Input: part model. Units: mm. Frame: model coordinates. Face numbers are marked on the shaded views. A direction names the side the tool comes from. Round coordinates to 2 decimals unless told otherwise and drop trailing zeros. Loops run counter-clockwise (first coordinate to the right, second up) from the corner with the lowest first, then second, coordinate; pieces in that order, holes last. Notation, with made-up numbers: M 13.5,42.5 L 38.5,42.5 A16 ccw 38.5,67.5 Z; hole C 68.5,-18.5 d9. An arc over 180 degrees is marked long. Return JSON: item names as keys, results as strings. Group by question number.
1) Section A-A (x = 62.5). Output: boundary loops of the cut face in (y, z).
2) Section D-D (x = 96). Output: boundary loops of the cut face in (y, z).
3) Section B-B (y = 24.5). Output: boundary loops of the cut face in (x, z).
4) Access query for the marked faces 1, 2, 3, 4 and 5. Directions: +Z, -Z, +X, -X, +Y, -Y. A direction counts if a zero-diameter tool reaches every point of the face in a straight line with its end or side. Return the directions, or none.
5) Material intervals for line 1 (X direction, y = 26, z = 10); line 2 (Z direction, x = 25, y = 32); line 3 (X direction, y = 9.5, z = 17), sorted ascending. Write a range as from..to.
6) Mould query, pull axis Y, two halves, no side actions, for the marked faces 6, 7 and 8. Classes: +Y half, -Y half, draft (parallel to the pull), parting line (faces both ways), or undercut.
7) Contact query for flat-ended pins moving along their axis: P1, Ø8, axis at x = 125, z = 10, coming from the +Y side; P2, Ø3, axis at x = 144.5, z = 9.5, coming from the -Y side; P3, Ø5, axis at x = 73.5, y = 29, coming from the -Z side; P4, Ø6, axis at x = 76.5, z = 7, coming from the +Y side. Output: stop coordinate, or through.
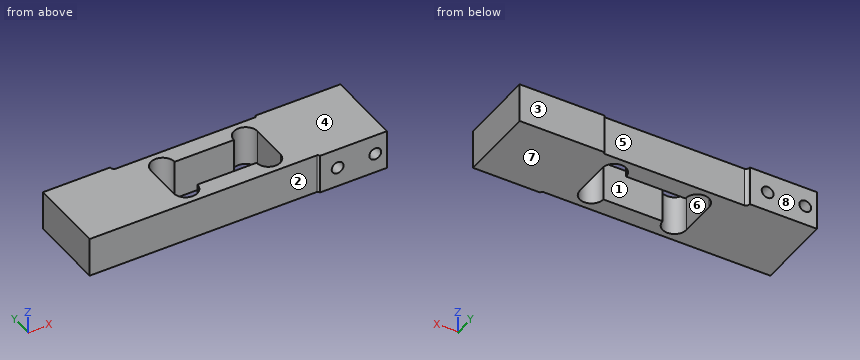
Autodesk Inventor part; units mm, degrees
ref_plane "YZ Plane" through (0, 0, 0) normal (1, 0, 0) x (0, 1, 0)
ref_plane "XZ Plane" through (0, 0, 0) normal (0, 1, 0) x (-1, 0, 0)
ref_plane "XY Plane" through (0, 0, 0) normal (0, 0, 1) x (1, 0, 0)
sketch "Sketch1" plane through (0, 0, 0) normal (0, 0, 1) x (1, 0, 0)
  line L0 (0, 0) -> (150, 0) construction
  line L1 (150, 0) -> (150, 39) construction
  line L2 (150, 39) -> (0, 39) construction
  line L3 (0, 38) -> (150, 38) construction
  line L4 (0, 37) -> (150, 37) construction
  arc A0 (106.25, 37) -> (107, 38) centre (106.0005, 37.9684) ccw
  arc A1 (34, 39) -> (35.5, 37) centre (35.999, 38.9367) ccw
  line L5 (0, -1) -> (150, -1) construction
  arc A2 (116, -1) -> (115.25, 0) centre (115.0005, -0.9684) ccw
  line L6 (75, 37) -> (75, 0) construction
  line L7 (0, 18.5) -> (150, 18.5) construction
  line L8 (75, 28) -> (60, 28)
  arc A3 (60, 28) -> (48, 28) centre (54, 28) ccw
  line L9 (48, 28) -> (48, 18.5)
  line L10 (75, 28) -> (90, 28)
  arc A4 (102, 28) -> (90, 28) centre (96, 28) ccw
  line L11 (102, 28) -> (102, 18.5)
  line L12 (75, 9) -> (60, 9)
  arc A5 (48, 9) -> (60, 9) centre (54, 9) ccw
  line L13 (48, 9) -> (48, 18.5)
  arc A6 (90, 9) -> (102, 9) centre (96, 9) ccw
  line L14 (75, 9) -> (90, 9)
  line L15 (102, 9) -> (102, 18.5)
  line L16 (0, 39) -> (0, 0)
  line L17 (115.25, 0) -> (0, 0)
  line L18 (116, -1) -> (150, -1)
  line L19 (150, -1) -> (150, 38)
  line L20 (150, 38) -> (107, 38)
  line L21 (106.25, 37) -> (35.5, 37)
  line L22 (34, 39) -> (0, 39)
  dimension "d0" = 150
  dimension "d1" = 39
  dimension "d9" = 34
  dimension "d11" = 1
  dimension "d17" = 1
  dimension "d18" = 43
  dimension "d19" = 1.25
  dimension "d20" = 1
  dimension "d21" = 2.5
  dimension "d22" = 2
  dimension "d23" = 1
  dimension "d24" = 34
  dimension "d25" = 1.25
  dimension "d26" = 1
  dimension "d27" = 15
  dimension "d29" = 12
  dimension "d30" = 6
extrude "Extrusion1" add sketch "Sketch1" along normal blind 20
sketch "Sketch2" plane through (116, -1, 0) normal (0, -1, 0) x (1, 0, 0)
  line L0 (0, 20) -> (34, 20) construction
  line L1 (0, 0) -> (34, 0) construction
  line L2 (34, 0) -> (34, 20) construction
  line L3 (34, 20) -> (0, 20) construction
  line L4 (0, 20) -> (0, 0) construction
  circle A0 centre (9, 10) radius 3
  circle A1 centre (28.05, 10) radius 3
  line L5 (-116, 0) -> (-116, 20) construction
  line L6 (34, 0) -> (0, 0) construction
  line L7 (-116, 20) -> (34, 20) construction
  line L8 (34, 20) -> (34, 0) construction
  line L9 (34, 0) -> (-116, 0) construction
  line L10 (-116, 0) -> (-116, 20) construction
  line L11 (-116, 20) -> (-0.75, 20) construction
  dimension "d33" = 6
  dimension "d34" = 10
  dimension "d35" = 25
  dimension "d36" = 6
  dimension "d37" = 19.05
extrude "Extrusion4" cut sketch "Sketch2" against normal blind 18
sketch "Sketch3" plane through (0, 39, 0) normal (0, 1, 0) x (1, 0, 0)
  line L0 (150, 0) -> (150, -20) construction
  line L1 (0, 0) -> (150, 0) construction
  line L2 (150, 0) -> (150, -20) construction
  line L3 (150, -20) -> (0, -20) construction
  line L4 (0, -20) -> (0, 0) construction
  circle A0 centre (5.95, -10) radius 3
  circle A1 centre (25, -10) radius 3
  dimension "d45" = 6
  dimension "d46" = 6
  dimension "d47" = 19.05
  dimension "d51" = 125
  dimension "d52" = 10
  dimension "d53" = 10
extrude "Extrusion5" cut sketch "Sketch3" against normal blind 18
thread "Thread1"
thread "Thread2"
thread "Thread3"
thread "Thread4"
equation "\"d0\" = lcl"
equation "\"d1\" = lch1"
equation "\"d9\" = lcwd2"
equation "\"d11\" = lch2 - lch1"
equation "\"d17\" = lch2 - lch1"
equation "\"d18\" = lcwd3"
equation "\"d23\" = lch2 - lch1"
equation "\"d24\" = lcwd2"
equation "\"d31\" = lcw"
equation "\"d33\" = dia1"
equation "\"d34\" = 0.5 * lcw"
equation "\"d35\" = lcwd1"
equation "\"d36\" = dia1"
equation "\"d37\" = lcsd"
equation "\"d43\" = td"
equation "\"d45\" = d48"
equation "\"d46\" = d48"
equation "\"d47\" = d49"
equation "\"d51\" = lcl - lcwd1"
equation "\"d52\" = 0.5 * lcw"
equation "\"d53\" = 0.5 * lcw"
equation "\"d54\" = td"
equation "\"dias\" = 8.8"
equation "\"stra1\" = 9.5"
equation "\"diab2\" = 6"
equation "\"stra\" = 25"
equation "\"db1\" = 6"
equation "\"ds1\" = 5.8"
equation "\"ds2\" = 1.6"
equation "\"ang\" = 120deg"
equation "\"db2\" = 3"
equation "\"diab3\" = 7"
equation "\"diab4\" = 3"
equation "\"dias1\" = 13.4375"
equation "\"dias3\" = 2"
equation "\"dias4\" = 4"
equation "\"t1\" = 3"
equation "\"t2\" = 3"
equation "\"t3\" = 6"
equation "\"t4\" = 6"
equation "\"t5\" = 3"
equation "\"diab1\" = 19"
equation "\"afw\" = 0.2"
equation "\"lcsd\" = 19.05"
equation "\"lcwd1\" = 25"
equation "\"lcwd2\" = 34"
equation "\"lcw\" = 20"
equation "\"lch1\" = 39"
equation "\"lch2\" = 40"
equation "\"lcl\" = 150"
equation "\"lcwd3\" = 43"
equation "\"dia1\" = 6"
equation "\"td\" = 18"
equation "\"d48\" = 6"
equation "\"d49\" = 19.05"
equation "\"bhh\" = 6"
equation "\"sw\" = 25"
equation "\"spacert\" = 2"
equation "\"sh\" = 31"
equation "\"pvct\" = 5"
equation "\"dia3\" = 8"
equation "\"dia4\" = 11"
equation "\"tankl\" = 379"
equation "\"play\" = 9"
equation "\"holeh\" = 26"
equation "\"surroundt\" = 5"
equation "\"slack\" = 0.5"
equation "\"play2\" = 3"
equation "\"diaoverflow\" = 25"
equation "\"diaph\" = 32"
equation "\"diawater\" = 25"
equation "\"diacucl\" = 32"
equation "\"diaair\" = 32"
equation "\"diasurroundhole\" = 42"
equation "\"diagrate\" = 12"
equation "\"gratespacing\" = 12.02082"
equation "\"bottomdist\" = 9.6355"
equation "\"sidedist\" = 13.9375"
equation "\"diahcl\" = 32"
equation "\"bracketwtop\" = 6"
equation "\"bracketwbottom\" = 6"
equation "\"nett\" = 1"
equation "\"nethole\" = 16"
equation "\"netside\" = 3.5"
equation "\"nettop\" = 7"
equation "\"netholespacing\" = 2"
equation "\"diaetape\" = 32"
properties part number "load cell" material "Aluminum 6061"
Returned:
{
 "1": {"outline": "M 0,0 L 9,0 L 9,20 L 0,20 Z; M 28,0 L 37,0 L 37,20 L 28,20 Z"},
 "2": {"outline": "M 0,0 L 3,0 L 3,20 L 0,20 Z; M 34,0 L 37,0 L 37,20 L 34,20 Z"},
 "3": {"outline": "M 0,0 L 48,0 L 48,20 L 0,20 Z; M 102,0 L 150,0 L 150,20 L 102,20 Z; hole C 5.95,10 d6; hole C 25,10 d6"},
 "4": {"face 1": "+Z, -Z", "face 2": "+Z, -Z, -X, -Y", "face 3": "+Z, -Z, +X, +Y", "face 4": "+Z, +X, -X, +Y, -Y", "face 5": "+Z, -Z, +Y"},
 "5": {"line 1": "x = 0..2.95, 8.95..22, 28..48, 102..150", "line 2": "z = 0..7, 13..20", "line 3": "x = 0..48, 102..150"},
 "6": {"face 6": "undercut", "face 7": "draft", "face 8": "+Y half"},
 "7": {"P1": "stops at y = 38", "P2": "stops at y = 17", "P3": "stops at z = 0", "P4": "stops at y = 37"}
}
